from build123d import *

# Parameters (mm, degrees)
SKETCH_1_R               = 11.555
EXTRUDE_1_DEPTH          = 11
CUT_EXTRUDE_1_DEPTH      = 11
PATTERN_CIRCULAR_1_COUNT = 25
SKETCH_3_R               = 14
EXTRUDE_2_DEPTH          = 1.5
SKETCH_4_R               = 9.5
EXTRUDE_3_DEPTH          = 10.5
CUT_EXTRUDE_START        = -9.5
CUT_EXTRUDE_2_DEPTH      = 0.5
CUT_EXTRUDE_3_REACH      = 26.5
SKETCH_6_R               = 4
CUT_EXTRUDE_4_REACH      = 26.5
CUT_EXTRUDE_6_DEPTH      = 0.75
CUT_EXTRUDE_6_DEPTH_BACK = 0.75


with BuildPart() as part:
    # Sketch 1 → Extrude 1 (new body)
    with BuildSketch(Plane.XY):
        Circle(SKETCH_1_R)
    extrude(amount=EXTRUDE_1_DEPTH)

    # Sketch 2 → Cut-Extrude 1 (cut)
    with BuildSketch(Plane.XY.offset(11)):
        with BuildLine():
            ThreePointArc((1.162550039, 11.496369097), (0, 11.555), (-1.162550039, 11.496369097))
            ThreePointArc((-1.162550039, 11.496369097), (-1.013703117, 11.389263051), (-0.955, 11.215536094))
            ThreePointArc((-0.955, 11.215536094), (0, 10.275), (0.955, 11.215536094))
            ThreePointArc((0.955, 11.215536094), (1.013703117, 11.389263051), (1.162550039, 11.496369097))
        make_face()
    cut_extrude_1 = extrude(amount=-CUT_EXTRUDE_1_DEPTH, mode=Mode.SUBTRACT)

    # Pattern Circular 1: Cut-Extrude 1 ×25 about axis
    pattern_circular_1_axis = Axis((0, 0, 0), (0, 0, 1))
    for i in range(1, PATTERN_CIRCULAR_1_COUNT):
        add(cut_extrude_1.rotate(pattern_circular_1_axis, i * 360 / PATTERN_CIRCULAR_1_COUNT), mode=Mode.SUBTRACT)

    # Sketch 3 → Extrude 2 (add)
    with BuildSketch(Plane.XY.offset(11)):
        Circle(SKETCH_3_R)
    extrude_2 = extrude(amount=EXTRUDE_2_DEPTH)

    # Mirror 1: Extrude 2 across plane
    add(extrude_2.mirror(Plane(origin=(0, 0, 5.5), x_dir=(1, 0, 0), z_dir=(0, 0, -1))))

    # Sketch 4 → Extrude 3 (add)
    with BuildSketch(Plane.XY.offset(12.5)):
        Circle(SKETCH_4_R)
    extrude(amount=EXTRUDE_3_DEPTH)

    # Sketch 5 → Cut-Extrude 2 (cut)
    with BuildSketch(Plane.XY.offset(23).offset(CUT_EXTRUDE_START)):
        with BuildLine():
            Line((-9.287087811, 2), (9.287087811, 2))
            ThreePointArc((9.287087811, 2), (0, -9.5), (-9.287087811, 2))
        make_face()
    extrude(amount=-CUT_EXTRUDE_2_DEPTH, mode=Mode.SUBTRACT)

    # Sketch 6 → Cut-Extrude 3 (cut, up to next)
    with BuildSketch(Plane.XY.offset(23), mode=Mode.PRIVATE) as cut_extrude_3_sk1:
        Circle(SKETCH_6_R)
    cut_extrude_3_tool1 = extrude(cut_extrude_3_sk1.sketch, amount=-CUT_EXTRUDE_3_REACH, mode=Mode.PRIVATE) & part.part
    add(cut_extrude_3_tool1.solids().sort_by_distance((0, 0, 23))[0], mode=Mode.SUBTRACT)

    # Sketch 7 → Cut-Extrude 4 (cut, up to next)
    with BuildSketch(Plane.XY.offset(23), mode=Mode.PRIVATE) as cut_extrude_4_sk1:
        with BuildLine():
            Line((-0.75, -3.929058411), (-0.75, -9.470348462))
            ThreePointArc((-0.75, -9.470348462), (0, -9.5), (0.75, -9.470348462))
            Line((0.75, -9.470348462), (0.75, -3.929058411))
            ThreePointArc((0.75, -3.929058411), (0, -4), (-0.75, -3.929058411))
        make_face()
    cut_extrude_4_tool1 = extrude(cut_extrude_4_sk1.sketch, amount=-CUT_EXTRUDE_4_REACH, mode=Mode.PRIVATE) & part.part
    add(cut_extrude_4_tool1.solids().sort_by_distance((0, -6.733246, 23))[0], mode=Mode.SUBTRACT)

    # Sketch 8 → Cut-Extrude 6 (cut, two sides)
    with BuildSketch(Plane(origin=(0, 0, 0), x_dir=(0, 0, -1), z_dir=(1, 0, 0))) as cut_extrude_6_sk:
        Polygon((-23, 7.5), (-18.5, 3.5), (-23, 3.5), align=None)
    extrude(amount=CUT_EXTRUDE_6_DEPTH, mode=Mode.SUBTRACT)
    extrude(cut_extrude_6_sk.sketch, amount=-CUT_EXTRUDE_6_DEPTH_BACK, mode=Mode.SUBTRACT)


solid = part.part
Source: CAD feature listing. Evaluate the final solid. Frame: model axes, mm. A direction names the side the tool comes from. Give positions to 0.01 mm unless a question says otherwise; leave off trailing zeros. Write each loop counter-clockwise with the first axis right and the second up, starting at its lowest first coordinate (ties: lowest second). Pieces come first, ordered by that corner, then holes. Notation, with made-up numbers: M 83,87 L 132,87 A19 cw 132,103 Z; hole C -28,15 d11. An arc over 180 degrees is marked long. Return JSON: item names as keys, results as strings. Group by question number.
1) Cut plane A-A, the plane x = 12. Output: boundary loops of the cut face in (y, z), plus the area to 3 significant figures.
2) Pin query (flat end, axial travel): P1, Ø1, axis at x = -11, z = 4.5, coming from the -Y side; P2, Ø8, axis at y = 5.5, z = 11.5, coming from the +X side; P3, Ø5, axis at y = -2, z = 16, coming from the -X side; P4, Ø7, axis at x = 0, y = 0, coming from the -Z side. Return the tip coordinate at first contact, or that it passes through.
3) Set-up query: faces 5 (the face through (6.06, -8.3, 5.58)), 6 (the face through (-0.75, -7, 18)), 7 (the face through (-3.3, -9.1, 12.5)). Return all of +Z, -Z, +X, -X, +Y, -Y with unobstructed straight access to the full face (end or side cutting, diameter ignored); none if empty.
4) Pull-direction query (Z, two-part tool) for faces 1 (the face through (0.75, -7, 18)), 2 (the face through (2.535, 9.958, 5.577)), 3 (the face through (3.802, -9.546, 5.577)), 4 (the face through (3, -3, -1.5)); classes: pulls with the +Z half, pulls with the -Z half, needs draft (parallel to the pull), parting line crosses it, or undercut.
5) Material intervals for line 1 along Z through (x, y) = (-4, -12); line 2 along Z through (x, y) = (7.5, -4); line 3 along X through (y, z) = (0, 6), sorted ascending. Write a range as [from, to].
6) Cut plane B-B, the plane y = -5.25. Output: boundary loops of the cut face in (x, z).
Recorded:
{
 "1": {"outline": "M -7.21,-1.5 L 7.21,-1.5 L 7.21,0 L -7.21,0 Z; M -7.21,11 L 7.21,11 L 7.21,12.5 L -7.21,12.5 Z", "area": "43.3 mm²"},
 "2": {"P1": "stops at y = -3.94", "P2": "stops at x = 13.92", "P3": "stops at x = -9.5", "P4": "passes through"},
 "3": {"face 5": "none", "face 6": "+Z, -Y", "face 7": "+Z"},
 "4": {"face 1": "needs draft", "face 2": "undercut", "face 3": "undercut", "face 4": "pulls with the -Z half"},
 "5": {"line 1": "z = [-1.5, 0], [11, 12.5]", "line 2": "z = [-1.5, 13], [13.5, 23]", "line 3": "x = [-10.56, -4], [4, 10.56]"},
 "6": {"outline": "M -12.98,-1.5 L 12.98,-1.5 L 12.98,0 L 9.33,0 L 9.33,11 L 12.98,11 L 12.98,12.5 L 7.92,12.5 L 7.92,13 L -7.92,13 L -7.92,12.5 L -12.98,12.5 L -12.98,11 L -9.33,11 L -9.33,0 L -12.98,0 Z; M -7.92,13.5 L -0.75,13.5 L -0.75,23 L -7.92,23 Z; M 0.75,13.5 L 7.92,13.5 L 7.92,23 L 0.75,23 Z"}
}
